```python
from build123d import *

# Parameters (mm, degrees)
BOSS_EXTRUDE1_DEPTH = 8
CUT_EXTRUDE1_REACH  = 17.62
SKETCH3_R           = 1.6
CUT_EXTRUDE2_DEPTH  = 4
FILLET1_R           = 3
SKETCH5_W           = 3
SKETCH5_H           = 2.5
CUT_EXTRUDE3_DEPTH  = 16.620499352


with BuildPart() as part:
    # Sketch1 → Boss-Extrude1 (new body)
    with BuildSketch(Plane.XY):
        with BuildLine():
            Line((-4, 0), (-12, 0))
            Line((-12, 0), (-12, 6))
            Line((-12, 6), (12, 6))
            Line((12, 6), (12, 0))
            Line((12, 0), (4, 0))
            ThreePointArc((4, 0), (0, 4), (-4, 0))
        make_face()
    extrude(amount=BOSS_EXTRUDE1_DEPTH)

    # Sketch3 → Cut-Extrude1 (cut, up to next)
    with BuildSketch(Plane.XZ, mode=Mode.PRIVATE) as cut_extrude1_sk1:
        with Locations((7, 4)):
            Circle(SKETCH3_R)
    cut_extrude1_tool1 = extrude(cut_extrude1_sk1.sketch, amount=-CUT_EXTRUDE1_REACH, mode=Mode.PRIVATE) & part.part
    # Sketch3 → Cut-Extrude1 (cut, up to next)
    with BuildSketch(Plane.XZ, mode=Mode.PRIVATE) as cut_extrude1_sk2:
        with Locations((-7, 4)):
            Circle(SKETCH3_R)
    cut_extrude1_tool2 = extrude(cut_extrude1_sk2.sketch, amount=-CUT_EXTRUDE1_REACH, mode=Mode.PRIVATE) & part.part
    add(cut_extrude1_tool1.solids().sort_by_distance((7, 0, 4))[0], mode=Mode.SUBTRACT)
    add(cut_extrude1_tool2.solids().sort_by_distance((-7, 0, 4))[0], mode=Mode.SUBTRACT)

    # Sketch4 → Cut-Extrude2 (cut)
    with BuildSketch(Plane(origin=(0, 6, 0), x_dir=(1, 0, 0), z_dir=(0, 1, 0))):
        Polygon((7, -0.420428331), (3.9, -2.210214166), (3.9, -5.789785834), (7, -7.579571669), (10.1, -5.789785834), (10.1, -2.210214166), align=None)
        Polygon((-7, -0.420428331), (-10.1, -2.210214166), (-10.1, -5.789785834), (-7, -7.579571669), (-3.9, -5.789785834), (-3.9, -2.210214166), align=None)
    extrude(amount=-CUT_EXTRUDE2_DEPTH, mode=Mode.SUBTRACT)

    # Fillet1
    fillet1_edges = [part.edges().sort_by_distance(p)[0] for p in [
        (12, 3, 8),
        (-12, 3, 8),
        (-12, 3, 0),
        (12, 3, 0),
    ]]
    fillet(fillet1_edges, radius=FILLET1_R)

    # Sketch5 → Cut-Extrude3 (cut, through all)
    with BuildSketch(Plane(origin=(0, 0, 0), x_dir=(-1, 0, 0), z_dir=(0, 0, -1))):
        with BuildLine():
            Line((-9, 6), (-9, 3.5))
            Line((-9, 3.5), (-4.873397172, 3.5))
            ThreePointArc((-4.873397172, 3.5), (-2.738612785, 5.338539127), (6e-09, 6))
            Line((6e-09, 6), (-9, 6))
        make_face()
        with Locations((-10.5, 4.75)):
            Rectangle(SKETCH5_W, SKETCH5_H)
        with BuildLine():
            Line((9, 6), (6e-09, 6))
            ThreePointArc((6e-09, 6), (2.73861279, 5.338539125), (4.873397172, 3.5))
            Line((4.873397172, 3.5), (9, 3.5))
            Line((9, 3.5), (9, 6))
        make_face()
        with Locations((10.5, 4.75)):
            Rectangle(SKETCH5_W, SKETCH5_H)
    extrude(amount=-CUT_EXTRUDE3_DEPTH, mode=Mode.SUBTRACT)


solid = part.part
```
CAD build for the part. Positions are in the model's coordinates, mm. A direction names the side the tool comes from. Coordinates: 2 decimals unless noted, no trailing zeros. Order: outer loops, then holes, each group sorted by start corner. A loop starts at its lowest first (then second) coordinate and runs counter-clockwise, first axis right, second up. Notation, with made-up numbers: (86, -10.75) - (139, -10.75) arc R15 ccw to (139, 9.25) - close; hole circle Ø11 at (26.25, 51). An arc over 180 degrees is marked (long way). Answer in a Markdown table with one row per item.
1. Slice it at D-D, the plane z = 5.25. List the corners of the cut face in (x, y).
Answer:
| item | result |
|---|---|
| outline | (-11.99, 0) - (-8, 0) - (-8, 2) - (-10.1, 2) - (-10.1, 3.5) - (-11.99, 3.5) - close; (-6, 0) - (-4, 0) arc R4 cw to (4, 0) - (6, 0) - (6, 2) - (3.9, 2) - (3.9, 4.56) arc R6 ccw to (-3.9, 4.56) - (-3.9, 2) - (-6, 2) - close; (8, 0) - (11.99, 0) - (11.99, 3.5) - (10.1, 3.5) - (10.1, 2) - (8, 2) - close |
2. Slice it at C-C, the plane x = -7.5. List the corners of the cut face in (y, z), then the cut area to 3 significant figures.
Answer:
| item | result |
|---|---|
| outline | (0, 0) - (3.5, 0) - (3.5, 0.71) - (2, 0.71) - (2, 2.48) - (0, 2.48) - close; (0, 5.52) - (2, 5.52) - (2, 7.29) - (3.5, 7.29) - (3.5, 8) - (0, 8) - close |
| area | 12.0 mm² |
3. Slice it at B-B, the plane z = 4. List the corners of the cut face in (x, y).
Answer:
| item | result |
|---|---|
| outline | (-12, 0) - (-8.6, 0) - (-8.6, 2) - (-10.1, 2) - (-10.1, 3.5) - (-12, 3.5) - close; (-5.4, 0) - (-4, 0) arc R4 cw to (4, 0) - (5.4, 0) - (5.4, 2) - (3.9, 2) - (3.9, 4.56) arc R6 ccw to (-3.9, 4.56) - (-3.9, 2) - (-5.4, 2) - close; (8.6, 0) - (12, 0) - (12, 3.5) - (10.1, 3.5) - (10.1, 2) - (8.6, 2) - close |
4. Slice it at A-A, the plane y = 1.25. List the corners of the cut face in (x, z), then the cut area to 3 significant figures.
Answer:
| item | result |
|---|---|
| outline | (-12, 3) arc R3 ccw to (-9, 0) - (-3.8, 0) - (-3.8, 8) - (-9, 8) arc R3 ccw to (-12, 5) - close; (3.8, 0) - (9, 0) arc R3 ccw to (12, 3) - (12, 5) arc R3 ccw to (9, 8) - (3.8, 8) - close; hole circle Ø3.2 at (-7, 4); hole circle Ø3.2 at (7, 4) |
| area | 107 mm² |
5. Drill centre lines: L1, parallel to Z at x = 7, y = 1.35; L2, parallel to X at y = 3.25, z = 2.25; L3, parallel to X at y = 3.25, z = 0.75. Where is each one in solid material? Low to high. Write a range as from..to.
Answer:
| item | result |
|---|---|
| L1 | 0..2.4, 5.6..8 |
| L2 | -11.9..-10.1, -3.9..-2.33, 2.33..3.9, 10.1..11.9 |
| L3 | -10.98..-7.57, -6.43..-2.33, 2.33..6.43, 7.57..10.98 |
6. 3-axis set-ups, long thin cutter, end or side, ignore diameter. For faces 1 (the face through (-11, 3.5, 4)), 2 (the face through (11, 3.5, 4)), 3 (the face through (8.528, 2.761, 6.697)): which of +Z, -Z, +X, -X, +Y, -Y reach the whole face in a straight line?
Answer:
| item | result |
|---|---|
| face 1 | +Z, -Z, -X, +Y |
| face 2 | +Z, -Z, +X, +Y |
| face 3 | +Y |
7. Pull direction Z, two halves, no side cores. Call faces 4 (the face through (0.1, 4.4, 0)), 5 (the face through (-8.572, 2.76, 6.672)), 6 (the face through (12, 2, 4)), 7 (the face through (5.472, 2.729, 1.303)): +Z half, -Z half, draft (parallel to the pull), parting line (faces both ways), or undercut.
Answer:
| item | result |
|---|---|
| face 4 | -Z half |
| face 5 | undercut |
| face 6 | draft |
| face 7 | undercut |
